```python
from build123d import *

# Parameters (mm, degrees)
BASPROSKE_W        = 3.175
BASPROSKE_H        = 13.758333333
TOOTHCUT_DEPTH     = 4.175
TEETHCUTS_COUNT    = 24
TEETHCUTS_ANGLE    = 345
CUT_EXTRUDE1_REACH = 5.175
CUT_EXTRUDE2_REACH = 5.175
SKETCH3_R          = 0.762


with BuildPart() as part:
    # BasProSke → Base-Revolve (revolve)
    with BuildSketch(Plane(origin=(0, 0, 0), x_dir=(1, 0, 0), z_dir=(0, 1, 0))):
        with Locations((1.5875, 6.879166667)):
            Rectangle(BASPROSKE_W, BASPROSKE_H)
    revolve(axis=Axis((-10, 0, 0), (1, 0, 0)))

    # TooCutSke → ToothCut (cut, through all)
    with BuildSketch(Plane(origin=(0, 0, 0), x_dir=(0, 0, -1), z_dir=(1, 0, 0))):
        with BuildLine():
            ThreePointArc((0.61154538, 11.362755163), (0, 11.3792), (-0.61154538, 11.362755163))
            ThreePointArc((-0.61154538, 11.362755163), (-0.876237748, 12.586912754), (-1.432393192, 13.709104797))
            ThreePointArc((-1.432393192, 13.709104797), (0, 13.783733333), (1.432393192, 13.709104797))
            ThreePointArc((1.432393192, 13.709104797), (0.876237748, 12.586912754), (0.61154538, 11.362755163))
        make_face()
    toothcut = extrude(amount=TOOTHCUT_DEPTH, mode=Mode.SUBTRACT)

    # TeethCuts: ToothCut ×24 about axis
    teethcuts_axis = Axis((-10, 0, 0), (1, 0, 0))
    for i in range(1, TEETHCUTS_COUNT):
        add(toothcut.rotate(teethcuts_axis, i * TEETHCUTS_ANGLE / (TEETHCUTS_COUNT - 1)), mode=Mode.SUBTRACT)

    # Sketch1 → Cut-Extrude1 (cut, up to next)
    with BuildSketch(Plane(origin=(3.175, 0, 0), x_dir=(0, 0, -1), z_dir=(1, 0, 0)), mode=Mode.PRIVATE) as cut_extrude1_sk1:
        with BuildLine():
            Line((-1.78325545, -2.35), (1.78325545, -2.35))
            ThreePointArc((1.78325545, -2.35), (0, 2.95), (-1.78325545, -2.35))
        make_face()
    cut_extrude1_tool1 = extrude(cut_extrude1_sk1.sketch, amount=-CUT_EXTRUDE1_REACH, mode=Mode.PRIVATE) & part.part
    add(cut_extrude1_tool1.solids().sort_by_distance((3.175, 0.146071, 0))[0], mode=Mode.SUBTRACT)

    # Sketch3 → Cut-Extrude2 (cut, up to next)
    with BuildSketch(Plane(origin=(3.175, 0, 0), x_dir=(0, 0, -1), z_dir=(1, 0, 0)), mode=Mode.PRIVATE) as cut_extrude2_sk1:
        with Locations((0, 4.7625)):
            Circle(SKETCH3_R)
    cut_extrude2_tool1 = extrude(cut_extrude2_sk1.sketch, amount=-CUT_EXTRUDE2_REACH, mode=Mode.PRIVATE) & part.part
    add(cut_extrude2_tool1.solids().sort_by_distance((3.175, 4.7625, 0))[0], mode=Mode.SUBTRACT)
    # Sketch3 → Cut-Extrude2 (cut, up to next)
    with BuildSketch(Plane(origin=(3.175, 0, 0), x_dir=(0, 0, -1), z_dir=(1, 0, 0)), mode=Mode.PRIVATE) as cut_extrude2_sk2:
        with Locations((-4.7625, 0)):
            Circle(SKETCH3_R)
    cut_extrude2_tool2 = extrude(cut_extrude2_sk2.sketch, amount=-CUT_EXTRUDE2_REACH, mode=Mode.PRIVATE) & part.part
    add(cut_extrude2_tool2.solids().sort_by_distance((3.175, 0, 4.7625))[0], mode=Mode.SUBTRACT)
    # Sketch3 → Cut-Extrude2 (cut, up to next)
    with BuildSketch(Plane(origin=(3.175, 0, 0), x_dir=(0, 0, -1), z_dir=(1, 0, 0)), mode=Mode.PRIVATE) as cut_extrude2_sk3:
        with Locations((4.7625, 0)):
            Circle(SKETCH3_R)
    cut_extrude2_tool3 = extrude(cut_extrude2_sk3.sketch, amount=-CUT_EXTRUDE2_REACH, mode=Mode.PRIVATE) & part.part
    add(cut_extrude2_tool3.solids().sort_by_distance((3.175, 0, -4.7625))[0], mode=Mode.SUBTRACT)
    # Sketch3 → Cut-Extrude2 (cut, up to next)
    with BuildSketch(Plane(origin=(3.175, 0, 0), x_dir=(0, 0, -1), z_dir=(1, 0, 0)), mode=Mode.PRIVATE) as cut_extrude2_sk4:
        with Locations((0, -4.7625)):
            Circle(SKETCH3_R)
    cut_extrude2_tool4 = extrude(cut_extrude2_sk4.sketch, amount=-CUT_EXTRUDE2_REACH, mode=Mode.PRIVATE) & part.part
    add(cut_extrude2_tool4.solids().sort_by_distance((3.175, -4.7625, 0))[0], mode=Mode.SUBTRACT)


solid = part.part
```
The listing builds one solid part. Answer for the finished solid, in the listing's coordinates (mm). A direction names the side the tool comes from. Round coordinates to 2 decimals unless told otherwise and drop trailing zeros. Order: outer loops, then holes, each group sorted by start corner. A loop starts at its lowest first (then second) coordinate and runs counter-clockwise, first axis right, second up. Notation, with made-up numbers: (-35.5, -8.75) - (-14.5, -8.75) arc R20 ccw to (-14.5, 12.25) - close; hole circle Ø3 at (-25, -6.5). An arc over 180 degrees is marked (long way). Put each result on its own line as item: value. Start each with the question number.
(1) Straight lines are drawn through the part: probe 1 along Y at (x, z) = (2.4, 0); probe 2 along Z at (x, y) = (0.8, -0.25); probe 3 along Z at (x, y) = (2, -11.5). For each, find the intervals that lie inside material, in ascending order. Write a range as from..to.
(2) Given P1, Ø1.4, axis at y = -4.76, z = 0, coming from the +X side; P2, Ø1, axis at x = 0.5, y = -10.5, coming from the +Z side, each flat-ended and moving along its own axis, determine where each tip first touches the part or whether it passes through.
(3) Find section A-A (z = 0). State how many separate pieces and enclosed holes the cut face has, plus the area to 3 significant figures.
(4) For faces 5 (the cylindrical face through (1.565, 5.535, -11.342)), 6 (the cylindrical face through (1.565, -4.106, -11.934)), 7 (the cylindrical face through (1.57, -4.09, 11.91)), determine the directions among +Z, -Z, +X, -X, +Y, -Y from which every point of the face is accessible in a straight line to the end or side of a thin tool.
(5) Determine the mould class of faces 1 (the cylindrical face through (1.57, -2.41, 12.39)), 2 (the cylindrical face through (1.565, 4.106, 11.934)), 3 (the cylindrical face through (1.565, -8.267, -9.491)), 4 (the cylindrical face through (1.57, -0.01, -11.38)) for opening direction Z: released by +Z, released by -Z, zero draft, split by the parting line, or undercut.
(6) Find section C-C (z = 4.5). Give the vertices of the cut face in (x, y) (3 decimals), plus the area to 3 significant figures.
Reply:
1. probe 1: -11.38..-5.52, -4..-2.35, 2.95..4, 5.52..11.38
1. probe 2: -11.38..-5.48, -4.04..-2.94, 2.94..4.04, 5.48..11.38
1. probe 3: -5.56..-3.84, -2.4..-0.63, 0.63..2.4, 3.84..5.56
2. P1: through
2. P2: z = 8.68
3. separate pieces: 4
3. enclosed holes: 0
3. area: 45.8 mm^2
4. face 5: +X, -X
4. face 6: -Z, +X, -X
4. face 7: +Z, +X, -X
5. face 1: undercut
5. face 2: released by +Z
5. face 3: undercut
5. face 4: released by -Z
6. outline: (0, -12.439) - (3.175, -12.439) - (3.175, -0.715) - (0, -0.715) - close; (0, 0.715) - (3.175, 0.715) - (3.175, 12.439) - (0, 12.439) - close
6. area: 74.4 mm^2
